The drawing under review shows one solid part. Ordinate dimensions are in mm from its lowest x, y, z. Give positions to 0.01 mm unless a question says otherwise; leave off trailing zeros. Loops run counter-clockwise (first coordinate to the right, second up) from the corner with the lowest first, then second, coordinate; pieces in that order, holes last. Notation, with made-up numbers: (46, 41) -> (88, 41) arc R24 ccw to (88, 78) -> close; hole circle Ø10 at (65, 51). An arc over 180 degrees is marked (long way). Answer in a Markdown table with one row per item. Add a question column.
(1) Consider section C-C on x = 14. Write out the cut boundary in (y, z) (1 decimal), then the cut area to 3 significant figures.
(2) Consider section A-A on x = 25. Write out the cut boundary in (y, z) (1 decimal), then the cut area to 3 significant figures.
(3) For line 1 (Y direction, x = 5, z = 3.5) (1 decimal); line 2 (X direction, y = 12.5, z = 3.25) (1 decimal); line 3 (Y direction, x = 11, z = 1.5) (1 decimal), list the stretches that pass through material, from the lowest coordinate up.
(4) Consider section B-B on z = 4. Count the separate pieces of the cut face and the enclosed holes in it, then the cut area to 3 significant figures.
(5) Consider section D-D on x = 20.5. Write out the cut boundary in (y, z).
(6) For pin 1 (2 mm diameter, centred on x = 5.77, y = 58.64, fed in from -Z), flat-tipped, find the tip position at first contact; note if it passes through.
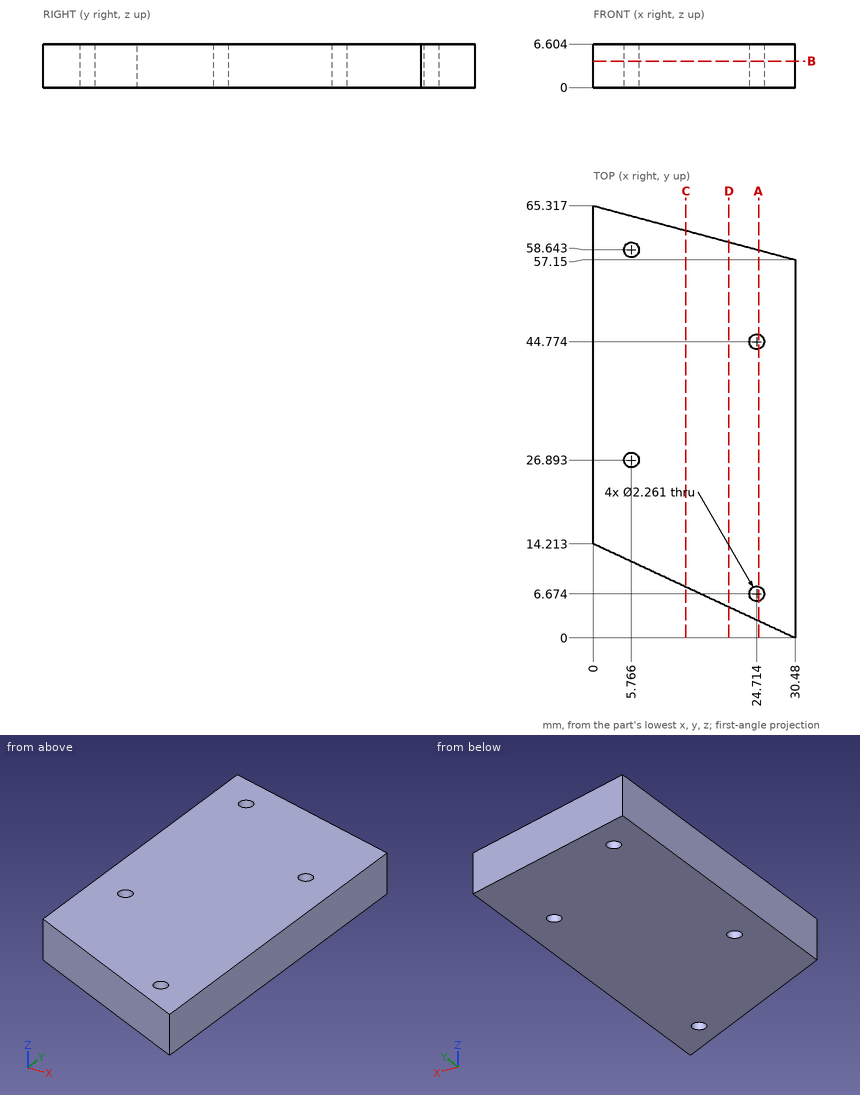
Values follow:
| question | item | result |
|---|---|---|
| 1 | outline | (7.7, 0) -> (61.6, 0) -> (61.6, 6.6) -> (7.7, 6.6) -> close |
| 1 | area | 356 mm2 |
| 2 | outline | (2.6, 0) -> (5.6, 0) -> (5.6, 6.6) -> (2.6, 6.6) -> close; (7.8, 0) -> (43.7, 0) -> (43.7, 6.6) -> (7.8, 6.6) -> close; (45.9, 0) -> (58.6, 0) -> (58.6, 6.6) -> (45.9, 6.6) -> close |
| 2 | area | 341 mm2 |
| 3 | line 1 | 11.9 to 26.1, 27.7 to 57.8, 59.5 to 64 |
| 3 | line 2 | 3.7 to 30.5 |
| 3 | line 3 | 9.1 to 62.4 |
| 4 | separate pieces | 1 |
| 4 | enclosed holes | 4 |
| 4 | area | 1,630 mm2 |
| 5 | outline | (4.65, 0) -> (59.82, 0) -> (59.82, 6.6) -> (4.65, 6.6) -> close |
| 6 | pin 1 | through |
